```python
from build123d import *

# Parameters (mm, degrees)
SKETCH3_R           = 0.6
SKETCH3_R_2         = 0.45
SKETCH3_R_3         = 2.425
BOSS_EXTRUDE1_DEPTH = 2


with BuildPart() as part:
    # Sketch2 → Revolve1 (revolve)
    with BuildSketch(Plane.XY):
        Polygon((2.25, 2), (2.25, 1.2), (1.125, 1.2), (1.125, 0.45), (2.425, 0.45), (2.425, -2), (3.6, -2), (3.6, 2), align=None)
    revolve(axis=Axis((0, 55, 0), (0, -1, 0)))

    # Sketch3 → Boss-Extrude1 (add)
    with BuildSketch(Plane(origin=(0, 0, 0), x_dir=(1, 0, 0), z_dir=(0, 1, 0))):
        with BuildLine():
            Line((0.190654206, -3.594947979), (16.195638629, -2.746140818))
            ThreePointArc((16.195638629, -2.746140818), (18.8, 0), (16.195638629, 2.746140818))
            Line((16.195638629, 2.746140818), (0.190654206, 3.594947979))
            ThreePointArc((0.190654206, 3.594947979), (0, 3.6), (-0.190654206, 3.594947979))
            Line((-0.190654206, 3.594947979), (-16.195638629, 2.746140818))
            ThreePointArc((-16.195638629, 2.746140818), (-18.8, 0), (-16.195638629, -2.746140818))
            Line((-16.195638629, -2.746140818), (-0.190654206, -3.594947979))
            ThreePointArc((-0.190654206, -3.594947979), (0, -3.6), (0.190654206, -3.594947979))
        make_face()
        with Locations((-16.75, 0)):
            Circle(SKETCH3_R, mode=Mode.SUBTRACT)
        with Locations((16.75, 0)):
            Circle(SKETCH3_R, mode=Mode.SUBTRACT)
        with Locations((-14, 0)):
            Circle(SKETCH3_R, mode=Mode.SUBTRACT)
        with Locations((14, 0)):
            Circle(SKETCH3_R, mode=Mode.SUBTRACT)
        with Locations((-12, 0)):
            Circle(SKETCH3_R_2, mode=Mode.SUBTRACT)
        with Locations((-10, 0)):
            Circle(SKETCH3_R_2, mode=Mode.SUBTRACT)
        with Locations((-8, 0)):
            Circle(SKETCH3_R_2, mode=Mode.SUBTRACT)
        with Locations((-6, 0)):
            Circle(SKETCH3_R_2, mode=Mode.SUBTRACT)
        with Locations((6, 0)):
            Circle(SKETCH3_R_2, mode=Mode.SUBTRACT)
        with Locations((8, 0)):
            Circle(SKETCH3_R_2, mode=Mode.SUBTRACT)
        with Locations((10, 0)):
            Circle(SKETCH3_R_2, mode=Mode.SUBTRACT)
        with Locations((12, 0)):
            Circle(SKETCH3_R_2, mode=Mode.SUBTRACT)
        Circle(SKETCH3_R_3, mode=Mode.SUBTRACT)
    extrude(amount=BOSS_EXTRUDE1_DEPTH)


solid = part.part
```
Check sheet for the modelled part. Datum: model origin and axes. Units: mm. A direction names the side the tool comes from. Coordinates: 2 decimals unless noted, no trailing zeros. Order: outer loops, then holes, each group sorted by start corner. A loop starts at its lowest first (then second) coordinate and runs counter-clockwise, first axis right, second up. Notation, with made-up numbers: M -11.75,36.5 L 43.25,36.5 A17 ccw 43.25,55.5 Z; hole C -27,-30.75 d4. An arc over 180 degrees is marked long. One line per question, with ' | ' between items. Start each with the question number.
Item 1: Sectioned sample at C-C on y = -0.85. Record the cut outline in (x, z) (3 decimals), and give its area (3 significant figures).
Item 2: Sectioned sample at B-B on x = 12. Record the cut outline in (y, z), and give its area (3 significant figures).
Item 3: Sectioned sample at A-A on x = -16.75. Record the cut outline in (y, z).
Item 4: Access from +Z, -Z, +X, -X, +Y, -Y to the whole of each face (thin tool, end or side, straight path). Record for faces 1 (the cylindrical face through (2.313, -0.792, 0.728)), 2 (the flat face through (-8.305, 0.986, 3.165)), 3 (the flat face through (-1, 1.2, 1)).
Item 5: Gauge pin test, flat ends, axial feed: P1, Ø1.4, axis at x = 16.75, z = 0, coming from the +Y side; P2, Ø4, axis at x = 8.5, z = -0.5, coming from the -Y side; P3, Ø1, axis at x = 7, y = 0.5, coming from the -Z side; P4, Ø1.3, axis at x = 0, z = 0, coming from the -Y side. Record the tip position at first contact, or that the pin passes through.
Item 6: Material ranges on line 1 (X direction, y = -0.45, z = 1.5); line 2 (Z direction, x = -0.5, y = -0.75); line 3 (Y direction, x = -14, z = -1.5), recorded low to high.
Item 7: Mould release check, pull along X, two halves, no side actions. Record for faces 4 (the cylindrical face through (-16.196, 0.986, 0.23)), 5 (the flat face through (8.081, 0.986, 3.176)), 6 (the cylindrical face through (-13.446, 0.986, 0.23)), 7 (the flat face through (-8.081, 0.986, -3.176)): pulls with the +X half, pulls with the -X half, needs draft (parallel to the pull), parting line crosses it, or undercut.
Answer below:
1) outline: C 0,0 d7.2; hole C 0,0 d4.85 | area: 22.2 mm^2
2) outline: M 0,-2.97 L 2,-2.97 L 2,-0.45 L 0,-0.45 Z; M 0,0.45 L 2,0.45 L 2,2.97 L 0,2.97 Z | area: 10.1 mm^2
3) outline: M 0,-2.66 L 2,-2.66 L 2,-0.6 L 0,-0.6 Z; M 0,0.6 L 2,0.6 L 2,2.66 L 0,2.66 Z
4) face 1: -Y | face 2: +Z, -X, +Y, -Y | face 3: +Y
5) P1: stops at y = 2 | P2: stops at y = 0 | P3: stops at z = -3.26 | P4: passes through
6) line 1: x = -3.27 to -1.91, 1.91 to 3.27 | line 2: z = -3.57 to -2.37, 2.37 to 3.57 | line 3: y = 0 to 2
7) face 4: undercut | face 5: pulls with the +X half | face 6: undercut | face 7: pulls with the -X half
